Part model, mm, in its own coordinate system. Round coordinates to 2 decimals unless told otherwise and drop trailing zeros. Loops run counter-clockwise (first coordinate to the right, second up) from the corner with the lowest first, then second, coordinate; pieces in that order, holes last.
from build123d import *

# Parameters (mm, degrees)
F0_W     = 254
F0_H     = 177.8
F0_R     = 63.5
F1_DEPTH = 127
F2_R     = 5.08
F3_R     = 12.7
F4_DEPTH = 127


with BuildPart() as f1:
    # F0 (on Top) → F1 (new body)
    with BuildSketch(Plane.XY):
        Rectangle(F0_W, F0_H)
        Circle(F0_R, mode=Mode.SUBTRACT)
    extrude(amount=F1_DEPTH)

    # F2
    f2_edges = [f1.edges().sort_by_distance(p)[0] for p in [
        (0, -88.9, 127),
        (127, 0, 127),
        (0, 88.9, 127),
        (-127, 0, 127),
        (-63.5, 0, 127),
        (-127, 88.9, 63.5),
        (-127, -88.9, 63.5),
        (-127, 0, 0),
        (127, -88.9, 63.5),
        (0, -88.9, 0),
        (127, 88.9, 63.5),
        (0, 88.9, 0),
    ]]
    fillet(f2_edges, radius=F2_R)

    # F3 (on face) → F4 (cut, through all)
    with BuildSketch(Plane.XY.offset(127)):
        with Locations((-101.6, 63.5)):
            Circle(F3_R)
        with Locations((101.6, 63.5)):
            Circle(F3_R)
        with Locations((101.6, -63.5)):
            Circle(F3_R)
        with Locations((-101.6, -63.5)):
            Circle(F3_R)
    extrude(amount=-F4_DEPTH, mode=Mode.SUBTRACT)


solid = f1.part
1) Slice it at C-C, the plane z = 107. Give the cut face in (x, y).
Values:
outline: (-127, -83.82) arc R5.08 ccw to (-121.92, -88.9) - (121.92, -88.9) arc R5.08 ccw to (127, -83.82) - (127, 83.82) arc R5.08 ccw to (121.92, 88.9) - (-121.92, 88.9) arc R5.08 ccw to (-127, 83.82) - close; hole circle Ø25.4 at (-101.6, -63.5); hole circle Ø25.4 at (-101.6, 63.5); hole circle Ø127 at (0, 0); hole circle Ø25.4 at (101.6, -63.5); hole circle Ø25.4 at (101.6, 63.5)
2) Slice it at B-B, the plane y = 0. Give the cut face in (x, z).
Values:
outline: (-127, 5.08) arc R5.08 ccw to (-121.92, 0) - (-63.5, 0) - (-63.5, 121.92) arc R5.08 ccw to (-68.58, 127) - (-121.92, 127) arc R5.08 ccw to (-127, 121.92) - close; (63.5, 0) - (127, 0) - (127, 121.92) arc R5.08 ccw to (121.92, 127) - (68.58, 127) arc R5.08 ccw to (63.5, 121.92) - close
3) Slice it at D-D, the plane x = 0. Give the cut face in (y, z).
Values:
outline: (-88.9, 5.08) arc R5.08 ccw to (-83.82, 0) - (-63.5, 0) - (-63.5, 121.92) arc R5.08 ccw to (-68.58, 127) - (-83.82, 127) arc R5.08 ccw to (-88.9, 121.92) - close; (63.5, 0) - (83.82, 0) arc R5.08 ccw to (88.9, 5.08) - (88.9, 121.92) arc R5.08 ccw to (83.82, 127) - (68.58, 127) arc R5.08 ccw to (63.5, 121.92) - close
4) Wall check: line 1 along Y through (x, z) = (101.6, 62); line 2 along Y through (x, z) = (0, 67); line 3 along X through (y, z) = (-56, 35.5). Give the ranges that are in metal, low to high.
Values:
line 1: y = -88.9 to -76.2, -50.8 to 50.8, 76.2 to 88.9
line 2: y = -88.9 to -63.5, 63.5 to 88.9
line 3: x = -127 to -111.85, -91.35 to -29.94, 29.94 to 91.35, 111.85 to 127
5) Slice it at A-A, the plane x = -101.6. Give the cut face in (y, z), then the cut area to 3 significant figures.
Values:
outline: (-88.9, 5.08) arc R5.08 ccw to (-83.82, 0) - (-76.2, 0) - (-76.2, 127) - (-83.82, 127) arc R5.08 ccw to (-88.9, 121.92) - close; (-50.8, 0) - (50.8, 0) - (50.8, 127) - (-50.8, 127) - close; (76.2, 0) - (83.82, 0) arc R5.08 ccw to (88.9, 5.08) - (88.9, 121.92) arc R5.08 ccw to (83.82, 127) - (76.2, 127) - close
area: 16,100 mm2
6) Mould opens along Y. For faces 1 (the face through (-89.486, -59.685, 64.389)), 2 (the face through (-13.77, -61.99, 60.11)), 3 (the face through (125.472, -87.451, 61.813)), 4 (the face through (-2, 76, 127)) say: released by +Y, released by -Y, zero draft, split by the parting line, or undercut.
Values:
face 1: undercut
face 2: undercut
face 3: released by -Y
face 4: zero draft
